```python
from build123d import *

# Parameters (mm, degrees)
SKETCH1_R           = 2
BOSS_EXTRUDE1_DEPTH = 3


with BuildPart() as part:
    # Sketch1 → Boss-Extrude1 (new body)
    with BuildSketch(Plane.XY):
        Polygon((-17.171078522, 8.102088167), (16.942973826, 8.102088167), (16.942973826, -1.897911833), (57.947591884, -1.897911833), (57.947591884, 8.102088167), (92.052408116, 8.102088167), (92.052408116, -8.436191264), (82.530366353, -26.812061334), (82.530366353, -94.896180398), (-7.810969029, -94.825139281), (-7.70389138, -26.741104419), (-17.197021163, -8.350281515), align=None)
        Circle(SKETCH1_R, mode=Mode.SUBTRACT)
        with Locations((75, 0)):
            Circle(SKETCH1_R, mode=Mode.SUBTRACT)
    extrude(amount=BOSS_EXTRUDE1_DEPTH)


solid = part.part
```
Verification items for the finished model (mm, model axes). A direction names the side the tool comes from. Give positions to 0.01 mm unless a question says otherwise; leave off trailing zeros. Loops run counter-clockwise (first coordinate to the right, second up) from the corner with the lowest first, then second, coordinate; pieces in that order, holes last.
1. Section check D-D, the plane y = -75. Enter the section's corners in (x, z), then the cut area to 3 significant figures.
2. Section check B-B, the plane z = 1.45. Enter the section's corners in (x, y), then the cut area to 3 significant figures.
3. Set-up check for faces 4 (the flat face through (82.53, -60, 1)), 5 (the flat face through (16.943, 3, 1)), 6 (the flat face through (38, -43, 3)): record each of +Z, -Z, +X, -X, +Y, -Y from which the full face is reachable in a straight line by a thin tool's end or side.
4. Go/stop test with a flat-tipped pin: pin 1 Ø3.5 at (x, y) = (0, 0) entering from -Z. Record where the tip stops, or that it passes through.
5. Section check A-A, the plane x = 75. Enter the section's corners in (y, z).
6. Thickness scan on line 1 (Y direction, x = 75, z = 1.15); line 2 (Y direction, x = 0, z = 1.05); line 3 (Y direction, x = 44.5, z = 1.6). Record the ranges inside material, lowest first.
7. Mould release check, pull along X, two halves, no side actions. Record for faces 1 (the flat face through (57.948, 3, 1)), 2 (the flat face through (-12.384, -17.674, 1.479)), 3 (the flat face through (38, -43, 0)): released by +X, released by -X, zero draft, split by the parting line, or undercut.
8. Section check C-C, the plane y = 0. Enter the section's corners in (x, z), then the cut area to 3 significant figures.
Geometry says:
1. outline: (-7.78, 0) - (82.53, 0) - (82.53, 3) - (-7.78, 3) - close
1. area: 271 mm2
2. outline: (-17.2, -8.35) - (-7.7, -26.74) - (-7.81, -94.83) - (82.53, -94.9) - (82.53, -26.81) - (92.05, -8.44) - (92.05, 8.1) - (57.95, 8.1) - (57.95, -1.9) - (16.94, -1.9) - (16.94, 8.1) - (-17.17, 8.1) - close; hole circle Ø4 at (0, 0); hole circle Ø4 at (75, 0)
2. area: 9,350 mm2
3. face 4: +Z, -Z, +X, -Y
3. face 5: +Z, -Z, +Y
3. face 6: +Z, +X, -X, +Y, -Y
4. pin 1: passes through
5. outline: (-94.89, 0) - (-2, 0) - (-2, 3) - (-94.89, 3) - close; (2, 0) - (8.1, 0) - (8.1, 3) - (2, 3) - close
6. line 1: y = -94.89 to -2, 2 to 8.1
6. line 2: y = -94.83 to -2, 2 to 8.1
6. line 3: y = -94.87 to -1.9
7. face 1: undercut
7. face 2: released by -X
7. face 3: zero draft
8. outline: (-17.18, 0) - (-2, 0) - (-2, 3) - (-17.18, 3) - close; (2, 0) - (16.94, 0) - (16.94, 3) - (2, 3) - close; (57.95, 0) - (73, 0) - (73, 3) - (57.95, 3) - close; (77, 0) - (92.05, 0) - (92.05, 3) - (77, 3) - close
8. area: 181 mm2
